```python
from build123d import *

# Parameters (mm, degrees)
BOSS_EXTRU_1_DEPTH      = 10
ESQUISSE2_R             = 1.5
ENL_V_MAT_EXTRU_1_DEPTH = 10


with BuildPart() as part:
    # Esquisse1 → Boss.-Extru.1 (new body)
    with BuildSketch(Plane.XY):
        with BuildLine():
            Line((0, 0), (0, 15.1))
            Line((0, 15.1), (20, 15.1))
            Line((20, 15.1), (20, 0))
            Line((20, 0), (32, 0))
            Line((32, 0), (32, 5))
            Line((32, 5), (25, 5))
            Line((25, 5), (25, 18.1))
            ThreePointArc((25, 18.1), (24.414213562, 19.514213562), (23, 20.1))
            Line((23, 20.1), (-3, 20.1))
            ThreePointArc((-3, 20.1), (-4.414213562, 19.514213562), (-5, 18.1))
            Line((-5, 18.1), (-5, 5))
            Line((-5, 5), (-12, 5))
            Line((-12, 5), (-12, 0))
            Line((-12, 0), (0, 0))
        make_face()
    extrude(amount=BOSS_EXTRU_1_DEPTH)

    # Esquisse2 → Enlèv. mat.-Extru.1 (cut)
    with BuildSketch(Plane(origin=(0, 5, 0), x_dir=(1, 0, 0), z_dir=(0, 1, 0))):
        with Locations(Location((-8.5, -5, 0), (0, 0, 270))):
            Circle(ESQUISSE2_R)
        with Locations(Location((28.5, -5, 0), (0, 0, 180))):
            Circle(ESQUISSE2_R)
    extrude(amount=-ENL_V_MAT_EXTRU_1_DEPTH, mode=Mode.SUBTRACT)


solid = part.part
```
Design review of the part built by this model. Coordinates are the model's own, in mm. A direction names the side the tool comes from. Give positions to 0.01 mm unless a question says otherwise; leave off trailing zeros. Loops run counter-clockwise (first coordinate to the right, second up) from the corner with the lowest first, then second, coordinate; pieces in that order, holes last. Notation, with made-up numbers: (37.25, -40) -> (79.25, -40) arc R19 cw to (79.25, -22) -> close; hole circle Ø2 at (-16, -37). An arc over 180 degrees is marked (long way). One line per item, written item: value.
Q1. For L1, parallel to X at y = 13.75, z = 8.25; L2, parallel to Z at x = 28.5, y = 2.5; L3, parallel to X at y = 2.5, z = 2.5, list the stretches that pass through material, from the lowest coordinate up.
Numbers:
L1: x = -5 to 0, 20 to 25
L2: z = 0 to 3.5, 6.5 to 10
L3: x = -12 to 0, 20 to 32
Q2. Machinability: for faces 1 (the flat face through (25, 11, 5)), 2 (the flat face through (-5, 12, 5)), 3 (the flat face through (10, 15.1, 5)), which of the approach directions +Z, -Z, +X, -X, +Y, -Y give a long, thin tool a straight path to every point of the face, cutting with its end or side? Answer none if there is none.
Numbers:
face 1: +Z, -Z, +X, +Y
face 2: +Z, -Z, -X, +Y
face 3: +Z, -Z, -Y
Q3. For pin 1 Ø3 at (y, z) = (12.5, 2.5) entering from -X; pin 2 Ø5 at (y, z) = (13, 7.5) entering from +X; pin 3 Ø4 at (x, z) = (-8.5, 5) entering from +Y, all flat-tipped, find the tip position at first contact; note any pin that passes through.
Numbers:
pin 1: stops at x = -5
pin 2: stops at x = 25
pin 3: stops at y = 5
Q4. We need section A-A on y = 4.25. Give the boundary of the cut face in (x, z).
Numbers:
outline: (-12, 0) -> (0, 0) -> (0, 10) -> (-12, 10) -> close; (20, 0) -> (32, 0) -> (32, 10) -> (20, 10) -> close; hole circle Ø3 at (-8.5, 5); hole circle Ø3 at (28.5, 5)
Q5. Draft analysis for pull direction X (two halves, no side actions). For faces 4 (the flat face through (26, 0, 5)), 5 (the cylindrical face through (-4.4, 19.53, 4.93)), 6 (the cylindrical face through (30, 3, 5)), state which applies: pulls with the +X half, pulls with the -X half, needs draft (parallel to the pull), parting line crosses it, or undercut.
Numbers:
face 4: needs draft
face 5: pulls with the -X half
face 6: undercut
Q6. We need section D-D on x = -8.5. Give the boundary of the cut face in (y, z).
Numbers:
outline: (0, 0) -> (5, 0) -> (5, 3.5) -> (0, 3.5) -> close; (0, 6.5) -> (5, 6.5) -> (5, 10) -> (0, 10) -> close
Q7. We need section C-C on y = 13.25. Give the boundary of the cut face in (x, z).
Numbers:
outline: (-5, 0) -> (0, 0) -> (0, 10) -> (-5, 10) -> close; (20, 0) -> (25, 0) -> (25, 10) -> (20, 10) -> close
Q8. We need section B-B on z = 5. Give the boundary of the cut face in (x, y), and give its area (3 significant figures).
Numbers:
outline: (-12, 0) -> (-10, 0) -> (-10, 5) -> (-12, 5) -> close; (-7, 0) -> (0, 0) -> (0, 15.1) -> (20, 15.1) -> (20, 0) -> (27, 0) -> (27, 5) -> (25, 5) -> (25, 18.1) arc R2 ccw to (23, 20.1) -> (-3, 20.1) arc R2 ccw to (-5, 18.1) -> (-5, 5) -> (-7, 5) -> close; (30, 0) -> (32, 0) -> (32, 5) -> (30, 5) -> close
area: 339 mm^2
